Verification items for the finished model (mm, model axes). A direction names the side the tool comes from. Coordinates: 2 decimals unless noted, no trailing zeros. Order: outer loops, then holes, each group sorted by start corner. A loop starts at its lowest first (then second) coordinate and runs counter-clockwise, first axis right, second up. Notation, with made-up numbers: (80.25, -16.75) -> (96.25, -16.75) arc R3 ccw to (96.25, -11.75) -> close; hole circle Ø7 at (-27.5, -38). An arc over 180 degrees is marked (long way). Write each question's results on one line, items separated by ' | '. Start each with the question number.
(1) Go/stop test with flat-tipped pins: pin 1 (1.4 mm diameter, centred on x = 13.5, z = 3, fed in from -Y); pin 2 (1.4 mm diameter, centred on y = 1.5, z = 2.5, fed in from +X). Record where each tip stops, or that it passes through.
(2) Draft check along X on faces 4 (the flat face through (30, 2, 2)), 5 (the flat face through (48, 42, 0)), 6 (the flat face through (100, 2, 2)). Enter one of: +X half, -X half, draft (parallel to the pull), parting line (faces both ways), or undercut.
(3) Cross-section at A-A on x = 45. Enter the section's corners in (y, z), and give its area (3 significant figures).
(4) Cross-section at D-D on z = 1.55. Give the number of separate pieces and of enclosed holes in the cut face, and give its area (4 significant figures).
(5) Thickness scan on probe 1 along X at (y, z) = (78, 1.55); probe 2 along Y at (x, z) = (45, 1.15); probe 3 along X at (y, z) = (53.5, 2.5). Record the ranges inside material, lowest first. Write a range as [from, to].
(6) Set-up check for faces 1 (the flat face through (12, 24.75, 2)), 2 (the flat face through (102, 4.75, 2)), 3 (the flat face through (10, 2, 2)): record each of +Z, -Z, +X, -X, +Y, -Y from which the full face is reachable in a straight line by a thin tool's end or side.
(7) Cross-section at B-B on y = 30. Enter the section's corners in (x, z), and give its area (3 significant figures).
(8) Cross-section at C-C on y = 20. Enter the section's corners in (x, z), and give its area (3 significant figures).
```python
from build123d import *

# Parameters (mm, degrees)
SKETCH1_R           = 2.5
BOSS_EXTRUDE1_DEPTH = 4.75
SKETCH2_W           = 5
SKETCH2_H           = 4.75
SKETCH2_W_2         = 4.75
SKETCH2_H_2         = 10
CUT_EXTRUDE1_DEPTH  = 134.927452376
SKETCH3_R           = 1.5
CUT_EXTRUDE2_DEPTH  = 134.927452376
SKETCH4_W           = 35.5
SKETCH4_H           = 4.75
CUT_EXTRUDE3_DEPTH  = 10
CAVITY1_OUTLINE_R   = 1.5
CAVITY1_DEPTH       = 4.75


# Read off the part's stored shape, not the designer's step: Cavity1
with BuildPart() as part:
    # Sketch1 → Boss-Extrude1 (new body)
    with BuildSketch(Plane.XY):
        with BuildLine():
            Line((-9.685424338, 2.488484559), (5.386220056, 61.148792841))
            ThreePointArc((5.386220056, 61.148792841), (15.733633721, 76.897010412), (33.561388608, 83))
            Line((33.561388608, 83), (105, 83))
            Line((105, 83), (105, 0))
            Line((105, 0), (-10.324792855, 0))
            Line((-10.324792855, 0), (-9.685424338, 2.488484559))
        make_face()
        with Locations((33.561388608, 53.909722104)):
            Circle(SKETCH1_R, mode=Mode.SUBTRACT)
        with BuildLine():
            ThreePointArc((67.975974789, 4.760599446), (77.719162031, 13.288409394), (85.405906554, 23.707967867))
            ThreePointArc((85.405906554, 23.707967867), (80.896997447, 40.800941239), (63.804024076, 36.292032133))
            ThreePointArc((63.804024076, 36.292032133), (59.320089771, 30.213956356), (53.63656388, 25.239400554))
            ThreePointArc((53.63656388, 25.239400554), (50.566868781, 7.830294546), (67.975974789, 4.760599446))
        make_face(mode=Mode.SUBTRACT)
    extrude(amount=BOSS_EXTRUDE1_DEPTH)

    # Sketch2 → Cut-Extrude1 (cut, through all)
    with BuildSketch(Plane.XY.offset(4.75)):
        with Locations((12.5, 2.375)):
            Rectangle(SKETCH2_W, SKETCH2_H)
        with Locations((102.5, 2.375)):
            Rectangle(SKETCH2_W, SKETCH2_H)
        with Locations((27.5, 2.375)):
            Rectangle(SKETCH2_W, SKETCH2_H)
        with Locations((87.5, 2.375)):
            Rectangle(SKETCH2_W, SKETCH2_H)
        with Locations((102.625, 19.75)):
            Rectangle(SKETCH2_W_2, SKETCH2_H_2)
        with Locations((12.375, 19.75)):
            Rectangle(SKETCH2_W_2, SKETCH2_H_2)
    extrude(amount=-CUT_EXTRUDE1_DEPTH, mode=Mode.SUBTRACT)

    # Sketch3 → Cut-Extrude2 (cut, through all)
    with BuildSketch(Plane.XY.offset(4.75)):
        with Locations((95, 78)):
            Circle(SKETCH3_R)
        with Locations((45, 78)):
            Circle(SKETCH3_R)
    extrude(amount=-CUT_EXTRUDE2_DEPTH, mode=Mode.SUBTRACT)

    # Sketch4 → Cut-Extrude3 (cut)
    with BuildSketch(Plane.XY.offset(4.75)):
        with Locations((70, 80.625)):
            Rectangle(SKETCH4_W, SKETCH4_H)
    extrude(amount=-CUT_EXTRUDE3_DEPTH, mode=Mode.SUBTRACT)

    # Cavity1 outline → Cavity1 (cut)
    with BuildSketch(Plane.XY):
        with Locations((8.414860226, 52.844005613)):
            Circle(CAVITY1_OUTLINE_R)
    extrude(amount=CAVITY1_DEPTH, mode=Mode.SUBTRACT)


solid = part.part
```
Results are:
1) pin 1: stops at y = 4.75 | pin 2: stops at x = 100
2) face 4: undercut | face 5: draft | face 6: +X half
3) outline: (0, 0) -> (76.5, 0) -> (76.5, 4.75) -> (0, 4.75) -> close; (79.5, 0) -> (83, 0) -> (83, 4.75) -> (79.5, 4.75) -> close | area: 380 mm2
4) separate pieces: 1 | enclosed holes: 6 | area: 7,185 mm2
5) probe 1: x = [17.25, 43.5], [46.5, 93.5], [96.5, 105] | probe 2: y = [0, 76.5], [79.5, 83] | probe 3: x = [3.42, 7.07], [9.76, 31.1], [36.03, 105]
6) face 1: +Z, -Z | face 2: +Z, -Z, +X, -Y | face 3: +Z, -Z, -Y
7) outline: (-2.62, 0) -> (59.12, 0) -> (59.12, 4.75) -> (-2.62, 4.75) -> close; (87.1, 0) -> (105, 0) -> (105, 4.75) -> (87.1, 4.75) -> close | area: 378 mm2
8) outline: (-5.19, 0) -> (10, 0) -> (10, 4.75) -> (-5.19, 4.75) -> close; (14.75, 0) -> (49.35, 0) -> (49.35, 4.75) -> (14.75, 4.75) -> close; (83.06, 0) -> (100.25, 0) -> (100.25, 4.75) -> (83.06, 4.75) -> close | area: 318 mm2
